```python
from build123d import *

# Parameters (mm, degrees)
SKETCH1_R               = 6.5
SKETCH1_R_2             = 1.5
BOSS_EXTRUDE1_DEPTH     = 3.175
SKETCH2_W               = 13
SKETCH2_H               = 3.175
BOSS_EXTRUDE2_DEPTH     = 14
SKETCH3_R               = 1.5
CUT_EXTRUDE1_DEPTH      = 18
FILLET1_R               = 5
BOSS_EXTRUDE3_START     = -3.175
BOSS_EXTRUDE3_OUTLINE_R = 1.5
BOSS_EXTRUDE3_DEPTH     = 3.175
FILLET3_R               = 1
BOSS_EXTRUDE4_START     = -3.175
BOSS_EXTRUDE4_DEPTH     = 3.175
SKETCH6_R               = 1.5
CUT_EXTRUDE2_DEPTH      = 3.175
CHAMFER1_SIZE           = 4
FILLET4_R               = 2
CUT_EXTRUDE3_DEPTH      = 10
FILLET5_R               = 2
SKETCH8_R               = 1.5
BOSS_EXTRUDE5_DEPTH     = 3.175
CHAMFER2_SIZE           = 4
FILLET6_R               = 2
SKETCH9_R               = 1.5
CUT_EXTRUDE4_DEPTH      = 10
SKETCH9_3_W             = 16.093211202
SKETCH9_3_H             = 15.71695658
SKETCH9_3_R             = 1.5
SKETCH9_3_W_2           = 4.964902022
SKETCH9_3_H_2           = 7.25050354
BOSS_EXTRUDE6_DEPTH     = 3.175
CHAMFER3_SIZE           = 6.5
FILLET7_R               = 2


# Read off the part's stored shape, not the designer's step: Boss-Extrude3
with BuildPart() as part:
    # Sketch1 → Boss-Extrude1 (new body)
    # profile 1 of 2: a face of its own
    with BuildSketch(Plane.XY):
        Circle(SKETCH1_R)
        Circle(SKETCH1_R_2, mode=Mode.SUBTRACT)
    # profile 2 of 2: a face of its own
    with BuildSketch(Plane.XY):
        with BuildLine():
            Line((-6.5, 18), (-6.5, 0))
            ThreePointArc((-6.5, 0), (0, 6.5), (6.5, 0))
            Line((6.5, 0), (6.5, 18))
            Line((6.5, 18), (-6.5, 18))
        make_face()
    extrude(amount=BOSS_EXTRUDE1_DEPTH)

    # Sketch2 → Boss-Extrude2 (add)
    with BuildSketch(Plane.XY.offset(3.175)):
        with Locations((0, 16.4125)):
            Rectangle(SKETCH2_W, SKETCH2_H)
    extrude(amount=BOSS_EXTRUDE2_DEPTH)

    # Sketch3 → Cut-Extrude1 (cut)
    with BuildSketch(Plane(origin=(0, 18, 0), x_dir=(1, 0, 0), z_dir=(0, 1, 0))):
        with Locations(Location((0, -11.175, 0), (0, 0, 270))):
            Circle(SKETCH3_R)
    extrude(amount=-CUT_EXTRUDE1_DEPTH, mode=Mode.SUBTRACT)

    # Fillet1
    fillet1_edges = [part.edges().sort_by_distance(p)[0] for p in [
        (-6.5, 16.4125, 17.175),
        (6.5, 16.4125, 17.175),
    ]]
    fillet(fillet1_edges, radius=FILLET1_R)

    # Boss-Extrude3 outline → Boss-Extrude3 (add)
    with BuildSketch(Plane(origin=(0, 0, 0), x_dir=(-1, 0, 0), z_dir=(0, 0, -1)).offset(BOSS_EXTRUDE3_START)):
        with BuildLine():
            ThreePointArc((6.5, 0), (4.596194078, -4.596194078), (0, -6.5))
            Line((0, -6.5), (10, -6.5))
            ThreePointArc((10, -6.5), (16.239069091, 1.823188658), (6.5, 5.477225575))
            Line((6.5, 5.477225575), (6.5, 0))
        make_face()
        with Locations((10, 0)):
            Circle(BOSS_EXTRUDE3_OUTLINE_R, mode=Mode.SUBTRACT)
    extrude(amount=BOSS_EXTRUDE3_DEPTH)

    # Fillet3
    fillet3_edges = [part.edges().sort_by_distance(p)[0] for p in [
        (0, 14.825, 3.175),
        (0, 18, 0),
    ]]
    fillet(fillet3_edges, radius=FILLET3_R)

    # Sketch5 → Boss-Extrude4 (add)
    with BuildSketch(Plane(origin=(0, 0, 0), x_dir=(-1, 0, 0), z_dir=(0, 0, -1)).offset(BOSS_EXTRUDE4_START)):
        with BuildLine():
            Line((32.012922913, -6.5), (32.012922913, 11.5))
            Line((32.012922913, 11.5), (6.5, 11.5))
            Line((6.5, 11.5), (6.5, 5.477225575))
            ThreePointArc((6.5, 5.477225575), (16.239069091, 1.823188658), (10, -6.5))
            Line((10, -6.5), (32.012922913, -6.5))
        make_face()
    extrude(amount=BOSS_EXTRUDE4_DEPTH)

    # Sketch6 → Cut-Extrude2 (cut)
    with BuildSketch(Plane(origin=(0, 0, 0), x_dir=(-1, 0, 0), z_dir=(0, 0, -1))):
        with Locations((18.012922913, -2.5)):
            Circle(SKETCH6_R)
        with Locations((28.012922913, -2.5)):
            Circle(SKETCH6_R)
        with Locations((18.012922913, 7.5)):
            Circle(SKETCH6_R)
        with Locations((28.012922913, 7.5)):
            Circle(SKETCH6_R)
        with Locations((23.012922913, 2.5)):
            Circle(SKETCH6_R)
    extrude(amount=-CUT_EXTRUDE2_DEPTH, mode=Mode.SUBTRACT)

    # Chamfer1
    # the kernel refuses this chamfer: 4 mm, written as the material it adds along each edge
    with BuildSketch(Plane(origin=(-6.5, 11.5, 3.175), x_dir=(0.027495876610586053, 0.9996219169112968, 0), z_dir=(0, 0, -1))) as chamfer1_piece_1:
        Polygon((CHAMFER1_SIZE * 0.999621916911, -CHAMFER1_SIZE * 0.0274958766106), (-CHAMFER1_SIZE * 0.0274958766106, -CHAMFER1_SIZE * 0.999621916911), (0, 0), align=None)
    extrude(amount=3.175)

    # Fillet4
    fillet4_edges = [part.edges().sort_by_distance(p)[0] for p in [
        (-32.012922913, 11.5, 1.5875),
        (-32.012922913, -6.5, 1.5875),
    ]]
    fillet(fillet4_edges, radius=FILLET4_R)

    # Sketch7 → Cut-Extrude3 (cut)
    with BuildSketch(Plane(origin=(0, 0, 0), x_dir=(-1, 0, 0), z_dir=(0, 0, -1))):
        Polygon((-6.5, 0), (0, -6.5), (-6.5, -6.5), align=None)
    extrude(amount=-CUT_EXTRUDE3_DEPTH, mode=Mode.SUBTRACT)

    # Fillet5
    fillet5_edges = [part.edges().sort_by_distance(p)[0] for p in [
        (6.5, 0, 1.5875),
        (-10.5, 11.5, 1.5875),
        (-6.5, 15.5, 1.5875),
        (0, -6.5, 1.5875),
    ]]
    fillet(fillet5_edges, radius=FILLET5_R)

    # Sketch8 → Boss-Extrude5 (add)
    # profile 1 of 4: a face of its own
    with BuildSketch(Plane(origin=(0, 0, 0), x_dir=(-1, 0, 0), z_dir=(0, 0, -1))):
        with BuildLine():
            Line((14.012922913, 11.5), (14.012922913, -6.5))
            Line((14.012922913, -6.5), (30.012922913, -6.5))
            ThreePointArc((30.012922913, -6.5), (31.427136475, -5.914213562), (32.012922913, -4.5))
            Line((32.012922913, -4.5), (32.012922913, 9.5))
            ThreePointArc((32.012922913, 9.5), (31.427136475, 10.914213562), (30.012922913, 11.5))
            Line((30.012922913, 11.5), (14.012922913, 11.5))
        make_face()
        with Locations((18.012922913, -2.5)):
            Circle(SKETCH8_R, mode=Mode.SUBTRACT)
        with Locations((18.012922913, 7.5)):
            Circle(SKETCH8_R, mode=Mode.SUBTRACT)
        with Locations((23.012922913, 2.5)):
            Circle(SKETCH8_R, mode=Mode.SUBTRACT)
        with Locations((28.012922913, -2.5)):
            Circle(SKETCH8_R, mode=Mode.SUBTRACT)
        with Locations((28.012922913, 7.5)):
            Circle(SKETCH8_R, mode=Mode.SUBTRACT)
    # profile 2 of 4: a face of its own
    with BuildSketch(Plane(origin=(0, 0, 0), x_dir=(-1, 0, 0), z_dir=(0, 0, -1))):
        Polygon((14.012922913, 26.5), (14.012922913, 11.5), (30.012922913, 11.5), (32.012922913, 11.5), (32.012922913, 26.5), align=None)
    # profile 3 of 4: a face of its own
    with BuildSketch(Plane(origin=(0, 0, 0), x_dir=(-1, 0, 0), z_dir=(0, 0, -1))):
        with BuildLine():
            Line((32.012922913, 11.5), (30.012922913, 11.5))
            ThreePointArc((30.012922913, 11.5), (31.427136475, 10.914213562), (32.012922913, 9.5))
            Line((32.012922913, 9.5), (32.012922913, 11.5))
        make_face()
    # profile 4 of 4: a face of its own
    with BuildSketch(Plane(origin=(0, 0, 0), x_dir=(-1, 0, 0), z_dir=(0, 0, -1))):
        with BuildLine():
            ThreePointArc((32.012922913, -4.5), (31.427136475, -5.914213562), (30.012922913, -6.5))
            Line((30.012922913, -6.5), (32.012922913, -6.5))
            Line((32.012922913, -6.5), (32.012922913, -4.5))
        make_face()
    extrude(amount=-BOSS_EXTRUDE5_DEPTH)

    # Chamfer2
    # the kernel refuses this chamfer: 4 mm, written as the material it adds along each edge
    with BuildSketch(Plane(origin=(-14.012922913, 11.5, 0), x_dir=(-0.027495876610586053, 0.9996219169112968, 0), z_dir=(0, 0, 1))) as chamfer2_piece_1:
        Polygon((CHAMFER2_SIZE * 0.999621916911, -CHAMFER2_SIZE * 0.0274958766106), (-CHAMFER2_SIZE * 0.0274958766106, -CHAMFER2_SIZE * 0.999621916911), (0, 0), align=None)
    extrude(amount=3.175)

    # Fillet6
    fillet6_edges = [part.edges().sort_by_distance(p)[0] for p in [
        (-32.012922913, 26.5, 1.5875),
        (-14.012922913, 26.5, 1.5875),
        (-14.012922913, 15.5, 1.5875),
        (-10.298499236, 11.785576323, 1.5875),
    ]]
    fillet(fillet6_edges, radius=FILLET6_R)

    # Sketch9 → Cut-Extrude4 (cut)
    with BuildSketch(Plane(origin=(0, 0, 0), x_dir=(-1, 0, 0), z_dir=(0, 0, -1))):
        with Locations((23.012922913, 19)):
            Circle(SKETCH9_R)
    extrude(amount=-CUT_EXTRUDE4_DEPTH, mode=Mode.SUBTRACT)

    # Sketch9<3> → Boss-Extrude6 (add)
    # profile 1 of 5: a face of its own
    with BuildSketch(Plane(origin=(0, 0, 0), x_dir=(-1, 0, 0), z_dir=(0, 0, -1))):
        with Locations((23.012922913, 2.5)):
            Rectangle(SKETCH9_3_W, SKETCH9_3_H)
        with Locations((28.012922913, -2.5)):
            Circle(SKETCH9_3_R, mode=Mode.SUBTRACT)
        with Locations((18.012922913, 7.5)):
            Circle(SKETCH9_3_R, mode=Mode.SUBTRACT)
        with Locations((18.012922913, -2.5)):
            Circle(SKETCH9_3_R, mode=Mode.SUBTRACT)
        with Locations((28.012922913, 7.5)):
            Circle(SKETCH9_3_R, mode=Mode.SUBTRACT)
        with Locations((23.012922913, 2.5)):
            Rectangle(SKETCH9_3_W_2, SKETCH9_3_H_2, mode=Mode.SUBTRACT)
    # profile 2 of 5: a face of its own
    with BuildSketch(Plane(origin=(0, 0, 0), x_dir=(-1, 0, 0), z_dir=(0, 0, -1))):
        with Locations((28.012922913, -2.5)):
            Circle(SKETCH9_3_R)
    # profile 3 of 5: a face of its own
    with BuildSketch(Plane(origin=(0, 0, 0), x_dir=(-1, 0, 0), z_dir=(0, 0, -1))):
        with Locations((28.012922913, 7.5)):
            Circle(SKETCH9_3_R)
    # profile 4 of 5: a face of its own
    with BuildSketch(Plane(origin=(0, 0, 0), x_dir=(-1, 0, 0), z_dir=(0, 0, -1))):
        with Locations((18.012922913, 7.5)):
            Circle(SKETCH9_3_R)
    # profile 5 of 5: a face of its own
    with BuildSketch(Plane(origin=(0, 0, 0), x_dir=(-1, 0, 0), z_dir=(0, 0, -1))):
        with Locations((18.012922913, -2.5)):
            Circle(SKETCH9_3_R)
    extrude(amount=-BOSS_EXTRUDE6_DEPTH)

    # Chamfer3
    chamfer3_edges = [part.edges().sort_by_distance(p)[0] for p in [
        (-32.012922913, -6.5, 1.5875),
    ]]
    chamfer(chamfer3_edges, length=CHAMFER3_SIZE)

    # Fillet7
    fillet7_edges = [part.edges().sort_by_distance(p)[0] for p in [
        (-25.512922913, -6.5, 1.5875),
        (-32.012922913, 0, 1.5875),
    ]]
    fillet(fillet7_edges, radius=FILLET7_R)


solid = part.part
```
Can you work these out from the model? Positions are in its coordinate system, mm. A direction names the side the tool comes from. Give positions to 0.01 mm unless a question says otherwise; leave off trailing zeros. Write each loop counter-clockwise with the first axis right and the second up, starting at its lowest first coordinate (ties: lowest second). Pieces come first, ordered by that corner, then holes. Notation, with made-up numbers: (-32.5, -34.5) -> (-15.5, -34.5) arc R12 cw to (-15.5, -11.5) -> close; hole circle Ø2 at (-23, 57.5). An arc over 180 degrees is marked (long way). One line per item, written item: value.
Q1. Imagine slicing it at B-B on x = 0. Please give me the cut outline in (y, z) (3 decimals), and give its area (3 significant figures).
Results found:
outline: (-6.32, 0) -> (-1.5, 0) -> (-1.5, 3.175) -> (-6.32, 3.175) -> close; (1.5, 0) -> (17, 0) arc R1 ccw to (18, 1) -> (18, 9.675) -> (14.825, 9.675) -> (14.825, 4.175) arc R1 cw to (13.825, 3.175) -> (1.5, 3.175) -> close; (14.825, 12.675) -> (18, 12.675) -> (18, 17.175) -> (14.825, 17.175) -> close
area: 103 mm^2
Q2. Which directions (+Z, -Z, +X, -X, +Y, -Y) give clear straight access to the entire face, cutting with the end or side of a thin tool? Please do faces 1 (the face through (-6.656, 15.553, 1.565)), 2 (the face through (-6.5, 16, 6)), 3 (the face through (-0.053, -6.344, 1.565)), 4 (the face through (0, 14.825, 9)), 5 (the face through (-0.091, 17.699, 0.285)).
Results found:
face 1: +Z, -Z, +Y
face 2: +Z, +Y
face 3: +Z, -Z, +X, -Y
face 4: +Z, +X, -X, -Y
face 5: -Z, +X, +Y
Q3. Imagine slicing it at A-A on y = 2.5. Please give me the cut outline in (x, z) (3 decimals).
Results found:
outline: (-32.013, 0) -> (-24.513, 0) -> (-24.513, 3.175) -> (-32.013, 3.175) -> close; (-21.513, 0) -> (6.5, 0) -> (6.5, 3.175) -> (-21.513, 3.175) -> close
Q4. Please list where these lines run through material, in increasing order: line 1 (X direction, y = 15, z = 11); line 2 (Z direction, x = -4, y = -2) (3 decimals); line 3 (Y direction, x = -10, z = 1.55). Write a range as [from, to].
Results found:
line 1: x = [-6.5, -1.49], [1.49, 6.5]
line 2: z = [0, 3.175]
line 3: y = [-6.5, -1.5], [1.5, 12.59]
Q5. We'd pull the mould along Y, two halves only. Please class faces 6 (the face through (-8, 14, 2)), 7 (the face through (-31.856, 0.053, 1.61)), 8 (the face through (-22.818, 20.487, 1.565)): +Y half, -Y half, draft (parallel to the pull), parting line (faces both ways), or undercut.
Results found:
face 6: +Y half
face 7: -Y half
face 8: undercut
Q6. For P1, Ø1, axis at y = 19.5, z = 1, coming from the +X side; P2, Ø2.5, axis at x = 0, z = 11.175, coming from the -Y side; P3, Ø3.5, axis at y = 15, z = 8.5, coming from the -X side; P4, Ø3.5, axis at x = -23.01, y = 2.5, coming from the +Z side (3 decimals), each with a flat end and sliding along its axis, tell me the tip position at first contact or that it passes through.
Results found:
P1: stops at x = -14.01
P2: passes through
P3: stops at x = -6.5
P4: stops at z = 3.175
Q7. Imagine slicing it at D-D on z = 2.5. Give the number of separate pieces and of enclosed holes in the cut face, and give its area (3 significant figures).
Results found:
separate pieces: 1
enclosed holes: 4
area: 992 mm^2
Q8. Imagine slicing it at C-C on y = 19. Please give me the cut outline in (x, z) (3 decimals).
Results found:
outline: (-32.013, 0) -> (-24.513, 0) -> (-24.513, 3.175) -> (-32.013, 3.175) -> close; (-21.513, 0) -> (-14.013, 0) -> (-14.013, 3.175) -> (-21.513, 3.175) -> close
